Could you check a few things on this model? Use its own coordinates, in mm. A direction names the side the tool comes from. Coordinates: 2 decimals unless noted, no trailing zeros. Loops run counter-clockwise (first coordinate to the right, second up) from the corner with the lowest first, then second, coordinate; pieces in that order, holes last.
from build123d import *

# Parameters (mm, degrees)
F0_W     = 54
F0_H     = 20
F1_DEPTH = 34
F2_W     = 50
F2_H     = 30
F3_DEPTH = 18
F5_W     = 5
F5_H     = 11
F6_DEPTH = 5
F7_R     = 1


with BuildPart() as f1:
    # F0 (on Front) → F1 (new body)
    with BuildSketch(Plane.XZ):
        with Locations((27, -10)):
            Rectangle(F0_W, F0_H)
    extrude(amount=F1_DEPTH)

    # F2 (on Top) → F3 (cut)
    with BuildSketch(Plane.XY):
        with Locations((27, -17)):
            Rectangle(F2_W, F2_H)
    extrude(amount=-F3_DEPTH, mode=Mode.SUBTRACT)

    # F5 (on offset) → F6 (cut)
    with BuildSketch(Plane(origin=(0, -32, 0), x_dir=(-1, 0, 0), z_dir=(0, 1, 0))):
        with Locations((-14.5, -10)):
            Rectangle(F5_W, F5_H)
        with Locations((-39.5, -9.9999997467)):
            Rectangle(F5_W, F5_H)
    extrude(amount=-F6_DEPTH, mode=Mode.SUBTRACT)

    # F7
    f7_edges = [f1.edges().sort_by_distance(p)[0] for p in [
        (54, -17, -20),
        (54, -17, 0),
        (54, 0, -10),
        (54, -34, -10),
        (27, 0, 0),
        (0, 0, -10),
        (27, 0, -20),
        (0, -17, 0),
        (0, -17, -20),
        (0, -34, -10),
    ]]
    fillet(f7_edges, radius=F7_R)


solid = f1.part
1) We'd pull the mould along X, two halves only. Please class faces 1 (the flat face through (27, 0, -10)), 2 (the flat face through (17, -33, -10)), 3 (the flat face through (0, -17, -10)), 4 (the flat face through (54, -17, -10)): released by +X, released by -X, zero draft, split by the parting line, or undercut.
2) If I drill on L1, parallel to Y at x = 25, z = -17.5; L2, parallel to X at y = -6, z = -9; L3, parallel to Z at x = 32, y = -16, over which ranges is the centre line in solid material (lowest first)?
3) Imagine slicing it at C-C on x = 25. List the corners of the cut face in (y, z) for me.
4) Will this pin go through, and if not, where does the flat tip stop? pin 1 (15 mm diameter, centred on x = 34.5, y = -10.5, fed in from +Z).
5) Imagine slicing it at A-A on x = 38.5. List the corners of the cut face in (y, z) for me.
6) Imagine slicing it at B-B on z = -7. List the corners of the cut face in (x, y) for me, plus the area to 3 significant figures.
7) Imagine slicing it at D-D on y = -15. List the corners of the cut face in (x, z) for me.
8) For faces 5 (the flat face through (21, -33, 0)), 6 (the flat face through (40, -33, -4.5)), 7 (the flat face through (27, -32, -9)), which set-ups out of +Z, -Z, +X, -X, +Y, -Y let a thin tool reach every point of the face, with its end or its side?
Solved:
1. face 1: zero draft
1. face 2: undercut
1. face 3: released by -X
1. face 4: released by +X
2. L1: y = -34 to -32, -2 to 0
2. L2: x = 0 to 2, 52 to 54
2. L3: z = -20 to -18
3. outline: (-34, -20) - (-1, -20) arc R1 ccw to (0, -19) - (0, -1) arc R1 ccw to (-1, 0) - (-2, 0) - (-2, -18) - (-32, -18) - (-32, 0) - (-34, 0) - close
4. pin 1: stops at z = -18
5. outline: (-34, -20) - (-1, -20) arc R1 ccw to (0, -19) - (0, -1) arc R1 ccw to (-1, 0) - (-2, 0) - (-2, -18) - (-32, -18) - (-32, -15.5) - (-34, -15.5) - close; (-34, -4.5) - (-32, -4.5) - (-32, 0) - (-34, 0) - close
6. outline: (0, -33) arc R1 ccw to (1, -34) - (12, -34) - (12, -32) - (2, -32) - (2, -2) - (52, -2) - (52, -32) - (42, -32) - (42, -34) - (53, -34) arc R1 ccw to (54, -33) - (54, -1) arc R1 ccw to (53, 0) - (1, 0) arc R1 ccw to (0, -1) - close; (17, -34) - (37, -34) - (37, -32) - (17, -32) - close
6. area: 315 mm2
7. outline: (0, -19) arc R1 ccw to (1, -20) - (53, -20) arc R1 ccw to (54, -19) - (54, -1) arc R1 ccw to (53, 0) - (52, 0) - (52, -18) - (2, -18) - (2, 0) - (1, 0) arc R1 ccw to (0, -1) - close
8. face 5: +Z, +X, -X, +Y, -Y
8. face 6: -Y
8. face 7: +Z
